Geometry check sheet. Reference: the model listing, model coordinates, mm. Face numbers are marked on the shaded views. A direction names the side the tool comes from. Round coordinates to 2 decimals unless told otherwise and drop trailing zeros. Loops run counter-clockwise (first coordinate to the right, second up) from the corner with the lowest first, then second, coordinate; pieces in that order, holes last. Notation, with made-up numbers: M 43.25,75 L 73.25,75 A26 cw 73.25,102 Z; hole C 53,89 d3. An arc over 180 degrees is marked long. Write item = value, one per line.
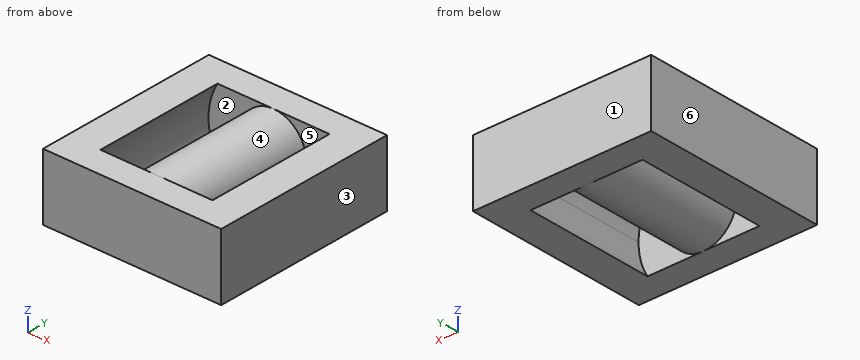
from build123d import *

# Parameters (mm, degrees)
BOSS_EXTRUDE1_DEPTH   = 62.4
SKETCH1_R             = 11.05
BOSS_EXTRUDE1_2_DEPTH = 62.4
BOSS_EXTRUDE1_3_DEPTH = 62.4
SKETCH2_W             = 59.8
SKETCH2_H             = 22.1
BOSS_EXTRUDE2_DEPTH   = 9.2
SKETCH3_W             = 59.8
SKETCH3_H             = 22.1
BOSS_EXTRUDE3_DEPTH   = 9.2


with BuildPart() as part:
    # Sketch1 → Boss-Extrude1 (new body)
    with BuildSketch(Plane(origin=(0, 0, 0), x_dir=(1, 0, 0), z_dir=(0, 1, 0))):
        with BuildLine():
            Line((-18.791953065, 11.05), (-29.9, 11.05))
            Line((-29.9, 11.05), (-29.9, -11.05))
            Line((-29.9, -11.05), (-18.791953065, -11.05))
            ThreePointArc((-18.791953065, -11.05), (-21.8, 0), (-18.791953065, 11.05))
        make_face()
    extrude(amount=BOSS_EXTRUDE1_DEPTH)



with BuildPart() as body_2:
    # Sketch1 → Boss-Extrude1 2 (new body)
    with BuildSketch(Plane(origin=(0, 0, 0), x_dir=(1, 0, 0), z_dir=(0, 1, 0))):
        Circle(SKETCH1_R)
    extrude(amount=BOSS_EXTRUDE1_2_DEPTH)


with BuildPart() as body_3:
    # Sketch1 → Boss-Extrude1 3 (new body)
    with BuildSketch(Plane(origin=(0, 0, 0), x_dir=(1, 0, 0), z_dir=(0, 1, 0))):
        with BuildLine():
            Line((29.9, 11.05), (18.791953065, 11.05))
            ThreePointArc((18.791953065, 11.05), (21.034549874, 5.7260555), (21.8, 0))
            ThreePointArc((21.8, 0), (21.034549874, -5.7260555), (18.791953065, -11.05))
            Line((18.791953065, -11.05), (29.9, -11.05))
            Line((29.9, -11.05), (29.9, 11.05))
        make_face()
    extrude(amount=BOSS_EXTRUDE1_3_DEPTH)


with BuildPart() as part_1:
    add(part.part)

    add(body_2.part)  # Boss-Extrude2 merges body 2

    add(body_3.part)  # Boss-Extrude2 merges body 3
    # Sketch2 → Boss-Extrude2 (add)
    with BuildSketch(Plane(origin=(0, 62.4, 0), x_dir=(1, 0, 0), z_dir=(0, 1, 0))):
        Rectangle(SKETCH2_W, SKETCH2_H)
    extrude(amount=-BOSS_EXTRUDE2_DEPTH)

    # Sketch3 → Boss-Extrude3 (add)
    with BuildSketch(Plane.XZ):
        Rectangle(SKETCH3_W, SKETCH3_H)
    extrude(amount=-BOSS_EXTRUDE3_DEPTH)


solid = part_1.part
(1) Sectioned sample at D-D on z = -1.5. Record the cut outline in (x, y).
Result set:
outline = M -29.9,0 L 29.9,0 L 29.9,62.4 L -29.9,62.4 Z; hole M -21.75,9.2 L -10.95,9.2 L -10.95,53.2 L -21.75,53.2 Z; hole M 10.95,9.2 L 21.75,9.2 L 21.75,53.2 L 10.95,53.2 Z
(2) Tool access check on the marked faces 1 and 2. Record the directions out of +Z, -Z, +X, -X, +Y, -Y that give a thin tool (end or side, any length) a straight path to the whole face; none if there is none.
Result set:
face_1 = +Z, -Z, +X, -X, +Y
face_2 = none
(3) Sectioned sample at A-A on y = 44.5. Record the cut outline in (x, z).
Result set:
outline = M -29.9,-11.05 L -18.79,-11.05 A21.8 cw -18.79,11.05 L -29.9,11.05 Z; C 0,0 d22.1; M 18.79,-11.05 L 29.9,-11.05 L 29.9,11.05 L 18.79,11.05 A21.8 cw Z
(4) Sectioned sample at B-B on x = -15. Record the cut outline in (y, z).
Result set:
outline = M 0,-11.05 L 9.2,-11.05 L 9.2,11.05 L 0,11.05 Z; M 53.2,-11.05 L 62.4,-11.05 L 62.4,11.05 L 53.2,11.05 Z
(5) Sectioned sample at C-C on z = -9.5. Record the cut outline in (x, y), then the cut area to 3 significant figures.
Result set:
outline = M -29.9,0 L 29.9,0 L 29.9,62.4 L -29.9,62.4 Z; hole M -19.62,9.2 L -5.64,9.2 L -5.64,53.2 L -19.62,53.2 Z; hole M 5.64,9.2 L 19.62,9.2 L 19.62,53.2 L 5.64,53.2 Z
area = 2,500 mm2
(6) Release check for a two-part mould opening along X. For the marked faces 3, 4, 5 and 6 record: released by +X, released by -X, zero draft, split by the parting line, or undercut.
Result set:
face_3 = released by +X
face_4 = undercut
face_5 = undercut
face_6 = released by -X
(7) Material ranges on line 1 along X through (y, z) = (24, 0.25); line 2 along X through (y, z) = (26, 7); line 3 along Y through (x, z) = (-12, 2.75), recorded low to high. Write a range as from..to.
Result set:
line_1 = -29.9..-21.8, -11.05..11.05, 21.8..29.9
line_2 = -29.9..-20.65, -8.55..8.55, 20.65..29.9
line_3 = 0..9.2, 53.2..62.4
(8) Depth check by flat-ended pin: pin 1 Ø10 at (x, y) = (7, 15.5) entering from +Z; pin 2 Ø2 at (x, y) = (10.5, 36) entering from -Z; pin 3 Ø4 at (x, y) = (-7.5, 23) entering from +Z. Enter the tip coordinate at first touch or a pass-through.
Result set:
pin_1 = 10.87
pin_2 = -5.64
pin_3 = 9.58
